Design review of the part built by this model. Coordinates are the model's own, in mm. Give positions to 0.01 mm unless a question says otherwise; leave off trailing zeros. Write each loop counter-clockwise with the first axis right and the second up, starting at its lowest first coordinate (ties: lowest second). Pieces come first, ordered by that corner, then holes. Notation, with made-up numbers: (14, 54) -> (50, 54) arc R38 ccw to (50, 92) -> close; hole circle Ø11 at (87.5, 84). An arc over 180 degrees is marked (long way). Answer as a JSON object with one key per item and string values.
```python
from build123d import *

# Parameters (mm, degrees)
BOSS_EXTRU_1_DEPTH           = 3
ENL_V_MAT_EXTRU_1_DEPTH      = 101.224747443
ENL_V_MAT_EXTRU_1_DEPTH_BACK = 101.224747443
ESQUISSE2_R                  = 2.75
CONG_1_R                     = 2


with BuildPart() as part:
    # Esquisse1 → Boss.-Extru.1 (new body)
    with BuildSketch(Plane.XY):
        Polygon((0, 0), (44, 0), (44, 15), (15, 90), (0, 90), align=None)
    extrude(amount=BOSS_EXTRU_1_DEPTH)

    # Esquisse2 → Enlèv. mat.-Extru.1 (cut, two sides: drawn at the far end of the back side and taken through both)
    with BuildSketch(Plane.XY.offset(3).offset(-ENL_V_MAT_EXTRU_1_DEPTH_BACK)):
        with Locations((7.5, 10)):
            Circle(ESQUISSE2_R)
        with Locations((7.5, 45)):
            Circle(ESQUISSE2_R)
        with Locations((7.5, 80)):
            Circle(ESQUISSE2_R)
        with Locations((22, 7.5)):
            Circle(ESQUISSE2_R)
        with Locations((38, 7.5)):
            Circle(ESQUISSE2_R)
    extrude(amount=ENL_V_MAT_EXTRU_1_DEPTH + ENL_V_MAT_EXTRU_1_DEPTH_BACK, mode=Mode.SUBTRACT)

    # Congé1
    cong_1_edges = [part.edges().sort_by_distance(p)[0] for p in [
        (0, 90, 1.5),
        (15, 90, 1.5),
        (44, 15, 1.5),
        (44, 0, 1.5),
        (0, 0, 1.5),
    ]]
    fillet(cong_1_edges, radius=CONG_1_R)


solid = part.part
```
(1) We need section A-A, the plane y = 45. State the section outline as (x, z) points, then the cut area to 3 significant figures.
Here are the results:
{"outline": "(0, 0) -> (4.75, 0) -> (4.75, 3) -> (0, 3) -> close; (10.25, 0) -> (32.4, 0) -> (32.4, 3) -> (10.25, 3) -> close", "area": "80.7 mm²"}
(2) We need section D-D, the plane x = 7.5. State the section outline as (y, z) points, then the cut area to 4 significant figures.
Here are the results:
{"outline": "(0, 0) -> (7.25, 0) -> (7.25, 3) -> (0, 3) -> close; (12.75, 0) -> (42.25, 0) -> (42.25, 3) -> (12.75, 3) -> close; (47.75, 0) -> (77.25, 0) -> (77.25, 3) -> (47.75, 3) -> close; (82.75, 0) -> (90, 0) -> (90, 3) -> (82.75, 3) -> close", "area": "220.5 mm²"}
(3) We need section B-B, the plane x = 38. State the section outline as (y, z) points.
Here are the results:
{"outline": "(0, 0) -> (4.75, 0) -> (4.75, 3) -> (0, 3) -> close; (10.25, 0) -> (30.52, 0) -> (30.52, 3) -> (10.25, 3) -> close"}
(4) The part is to be moulded in two halves that separate along X. For faces 1 (the flat face through (0, 46, 1)), 2 (the cylindrical face through (7.142, 47.727, 1.479)), 3 (the cylindrical face through (14.746, 89.659, 1.521)), say which applies: +X half, -X half, draft (parallel to the pull), parting line (faces both ways), or undercut.
Here are the results:
{"face 1": "-X half", "face 2": "undercut", "face 3": "+X half"}
(5) We need section C-C, the plane z = 1.3. State the section outline as (x, y) points.
Here are the results:
{"outline": "(0, 2) arc R2 ccw to (2, 0) -> (42, 0) arc R2 ccw to (44, 2) -> (44, 14.63) arc R2 ccw to (43.87, 15.35) -> (15.49, 88.72) arc R2 ccw to (13.63, 90) -> (2, 90) arc R2 ccw to (0, 88) -> close; hole circle Ø5.5 at (7.5, 10); hole circle Ø5.5 at (7.5, 45); hole circle Ø5.5 at (7.5, 80); hole circle Ø5.5 at (22, 7.5); hole circle Ø5.5 at (38, 7.5)"}
(6) For line 1 along Y through (x, z) = (7.5, 1.95); line 2 along Y through (x, z) = (9, 2.7); line 3 along X through (y, z) = (7.5, 2.2), list the stretches that pass through material, from the lowest coordinate up.
Here are the results:
{"line 1": "y = 0 to 7.25, 12.75 to 42.25, 47.75 to 77.25, 82.75 to 90", "line 2": "y = 0 to 7.7, 12.3 to 42.7, 47.3 to 77.7, 82.3 to 90", "line 3": "x = 0 to 6.35, 8.65 to 19.25, 24.75 to 35.25, 40.75 to 44"}
(7) Clearance check with flat-ended pins moving along their axes: pin 1 (5 mm diameter, centred on x = 7.5, y = 10, fed in from +Z); pin 2 (1 mm diameter, centred on y = 61.5, z = 1.5, fed in from +X). State where each tip first meets the part, or that it passes through.
Here are the results:
{"pin 1": "passes through", "pin 2": "stops at x = 26.21"}
